Study the drawing (mm; zero at the part's minimum x, y, z) and answer. A direction names the side the tool comes from. Round coordinates to 2 decimals unless told otherwise and drop trailing zeros. Loops run counter-clockwise (first coordinate to the right, second up) from the corner with the lowest first, then second, coordinate; pieces in that order, holes last. Notation, with made-up numbers: (86, -4) -> (126, -4) arc R25 ccw to (126, 10) -> close; hole circle Ø5 at (5, -11). An arc over 180 degrees is marked (long way). Write each question's results on one line, items separated by ' | '. Start each with the question number.
(1) Flat-ended cylindrical pins translate along their axes: pin 1 (4 mm diameter, centred on x = 29.5, y = 6, fed in from +Z) (3 decimals); pin 2 (3 mm diameter, centred on x = 22.5, z = 2, fed in from +Y); pin 3 (5 mm diameter, centred on y = 6, z = 10, fed in from -X); pin 4 (1 mm diameter, centred on x = 30, y = 9, fed in from -Z). Find the tip coordinate at first contact, or state that the pin passes through.
(2) Straight lines are drawn through the part: probe 1 along X at (y, z) = (11.5, 6); probe 2 along Y at (x, z) = (24, 7); probe 3 along Z at (x, y) = (10.5, 3.25). For each, find the intervals that lie inside material, in ascending order.
(3) For the marked faces 1 and 2, determine the directions among +Z, -Z, +X, -X, +Y, -Y from which every point of the face is accessible in a straight line to the end or side of a thin tool.
(4) The part is cut by section D-D (z = 1). Determine the outline of the cut face in (x, y), plus the area to 3 significant figures.
(5) The part is cut by section C-C (x = 4.5). Determine the outline of the cut face in (y, z) (3 decimals).
(6) The part is cut by section B-B (y = 9.75). Determine the outline of the cut face in (x, z).
(7) The part is cut by section A-A (z = 6.5). Determine the outline of the cut face in (x, y), plus the area to 3 significant figures.
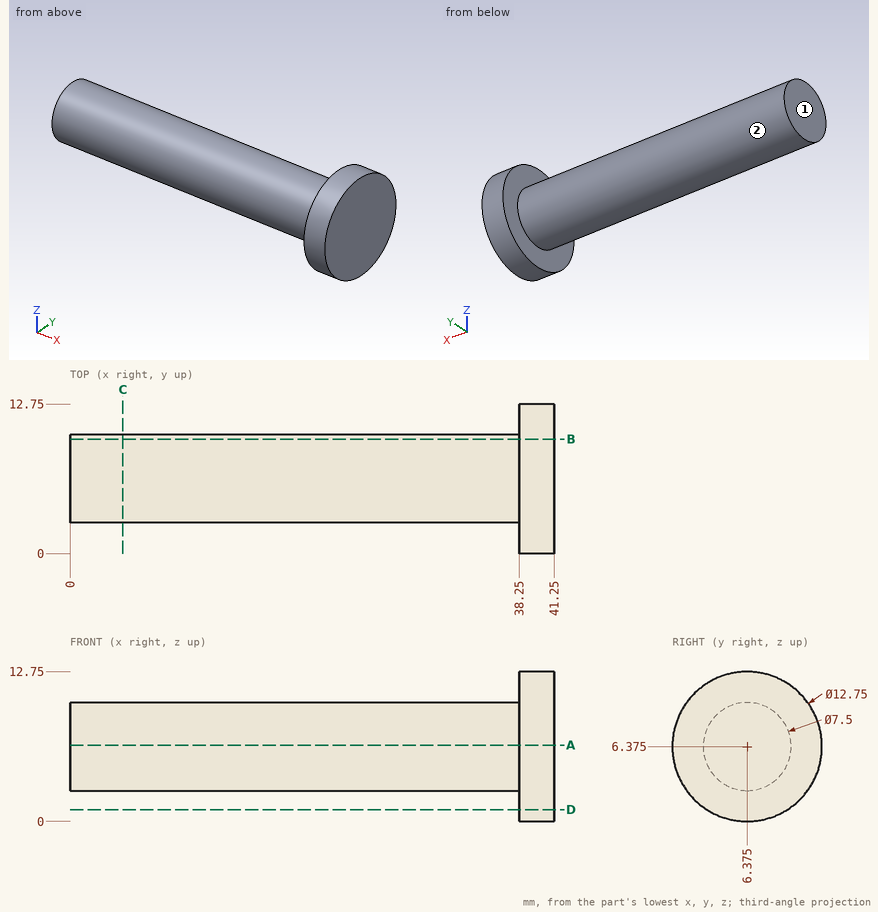
Checked values:
1) pin 1: stops at z = 10.125 | pin 2: stops at y = 8.78 | pin 3: stops at x = 0 | pin 4: stops at z = 3.29
2) probe 1: x = 38.25 to 41.25 | probe 2: y = 2.68 to 10.07 | probe 3: z = 4.3 to 8.45
3) face 1: +Z, -Z, -X, +Y, -Y | face 2: -X
4) outline: (38.25, 2.95) -> (41.25, 2.95) -> (41.25, 9.8) -> (38.25, 9.8) -> close | area: 20.6 mm2
5) outline: circle Ø7.5 at (6.375, 6.375)
6) outline: (0, 4.74) -> (38.25, 4.74) -> (38.25, 0.97) -> (41.25, 0.97) -> (41.25, 11.78) -> (38.25, 11.78) -> (38.25, 8.01) -> (0, 8.01) -> close
7) outline: (0, 2.63) -> (38.25, 2.63) -> (38.25, 0) -> (41.25, 0) -> (41.25, 12.75) -> (38.25, 12.75) -> (38.25, 10.12) -> (0, 10.12) -> close | area: 325 mm2
